from build123d import *

# Parameters (mm, degrees)
SKIZZE3_W                       = 11
SKIZZE3_H                       = 20
AUFSATZ_LINEAR_AUSTRAGEN1_DEPTH = 50
SKIZZE4_R                       = 2.375
SCHNITT_LINEAR_AUSTRAGEN1_DEPTH = 10
AUFSATZ_LINEAR_AUSTRAGEN2_DEPTH = 50
SKIZZE5_R                       = 2.3
SCHNITT_LINEAR_AUSTRAGEN2_DEPTH = 56.11862208
SKIZZE6_R                       = 3.75
SCHNITT_LINEAR_AUSTRAGEN3_DEPTH = 4.5
SKIZZE8_R                       = 4.25
SCHNITT_LINEAR_AUSTRAGEN4_DEPTH = 6.5
VERRUNDUNG1_R                   = 1
FASE1_SIZE                      = 0.75
VERRUNDUNG2_R                   = 2


with BuildPart() as part:
    # Skizze3 → Aufsatz-Linear austragen1 (new body)
    with BuildSketch(Plane.XY):
        with Locations((5.5, -10)):
            Rectangle(SKIZZE3_W, SKIZZE3_H)
    extrude(amount=-AUFSATZ_LINEAR_AUSTRAGEN1_DEPTH)

    # Skizze4 → Schnitt-Linear austragen1 (cut)
    with BuildSketch(Plane.ZY):
        with Locations(Location((-40, -7, 0), (0, 0, 270))):
            Circle(SKIZZE4_R)
        with Locations(Location((-10, -7, 0), (0, 0, 270))):
            Circle(SKIZZE4_R)
    extrude(amount=-SCHNITT_LINEAR_AUSTRAGEN1_DEPTH, mode=Mode.SUBTRACT)

    # Skizze7 → Aufsatz-Linear austragen2 (add)
    with BuildSketch(Plane.XY):
        Polygon((11, -13.5), (11, -6.5), (11.75, -7.25), (11.75, -12.75), align=None)
    extrude(amount=-AUFSATZ_LINEAR_AUSTRAGEN2_DEPTH)

    # Skizze5 → Schnitt-Linear austragen2 (cut, through all)
    with BuildSketch(Plane.ZY):
        with Locations(Location((-25, -10, 0), (0, 0, 270))):
            Circle(SKIZZE5_R)
    extrude(amount=-SCHNITT_LINEAR_AUSTRAGEN2_DEPTH, mode=Mode.SUBTRACT)

    # Skizze6 → Schnitt-Linear austragen3 (cut)
    with BuildSketch(Plane.ZY):
        with Locations(Location((-25, -10, 0), (0, 0, 270))):
            Circle(SKIZZE6_R)
    extrude(amount=-SCHNITT_LINEAR_AUSTRAGEN3_DEPTH, mode=Mode.SUBTRACT)

    # Skizze8 → Schnitt-Linear austragen4 (cut)
    with BuildSketch(Plane(origin=(11, 0, 0), x_dir=(0, 0, -1), z_dir=(1, 0, 0))):
        with Locations((25, -10)):
            Circle(SKIZZE8_R)
    extrude(amount=SCHNITT_LINEAR_AUSTRAGEN4_DEPTH, mode=Mode.SUBTRACT)

    # Verrundung1
    # the kernel refuses this fillet: 1 mm, written as the material it takes off along each edge
    with BuildSketch(Plane(origin=(11.75, -10, -25), x_dir=(0, 0.9561204309063354, -0.29297392649088017), z_dir=(0, 0.29297392649088017, 0.9561204309063354))) as verrundung1_piece_1:
        with BuildLine():
            CenterArc((5.218245837, 1), VERRUNDUNG1_R, 194.477512186, 75.522487814)
            Line((5.218245837, 0), (5.218245837, -0.02))
            Line((5.218245837, -0.02), (4.25, -0.02))
            Line((4.25, -0.02), (4.23, 0))
            ThreePointArc((4.23, 0), (4.23, 0.375), (4.230635083, 0.745))
            Line((4.230635083, 0.745), (4.25, 0.75))
        make_face()
    revolve(axis=Axis((11.75, -10, -25), (-1, 0, 0)), revolution_arc=145.927830349, mode=Mode.SUBTRACT)
    with BuildSketch(Plane(origin=(11.75, -10, -25), x_dir=(0, -0.9561204309062743, 0.292973926491079), z_dir=(0, -0.292973926491079, -0.9561204309062743))) as verrundung1_piece_2:
        with BuildLine():
            CenterArc((5.218245837, 1), VERRUNDUNG1_R, 194.477512186, 75.522487814)
            Line((5.218245837, 0), (5.218245837, -0.02))
            Line((5.218245837, -0.02), (4.25, -0.02))
            Line((4.25, -0.02), (4.23, 0))
            ThreePointArc((4.23, 0), (4.23, 0.375), (4.230635083, 0.745))
            Line((4.230635083, 0.745), (4.25, 0.75))
        make_face()
    revolve(axis=Axis((11.75, -10, -25), (-1, 0, 0)), revolution_arc=145.927830349, mode=Mode.SUBTRACT)

    # Fase1
    fase1_edges = [part.edges().sort_by_distance(p)[0] for p in [
        (5.5, -20, -50),
        (5.5, -20, 0),
        (5.5, 0, 0),
        (11, -20, -25),
        (0, -20, -25),
        (0, 0, -25),
        (11, 0, -25),
        (5.5, 0, -50),
    ]]
    chamfer(fase1_edges, length=FASE1_SIZE)

    # Verrundung2
    verrundung2_edges = [part.edges().sort_by_distance(p)[0] for p in [
        (11, -3.625, 0),
        (11, -3.625, -50),
        (11.375, -6.875, 0),
        (11.375, -13.125, 0),
        (11.75, -10, 0),
        (11.375, -6.875, -50),
        (11.75, -10, -50),
        (11.375, -13.125, -50),
        (0, -10, 0),
        (0, -10, -50),
        (11, -16.375, -50),
        (11, -16.375, 0),
    ]]
    fillet(verrundung2_edges, radius=VERRUNDUNG2_R)


solid = part.part
Input: part model. Units: mm. Frame: model coordinates. A direction names the side the tool comes from. Give positions to 0.01 mm unless a question says otherwise; leave off trailing zeros. Order: outer loops, then holes, each group sorted by start corner. A loop starts at its lowest first (then second) coordinate and runs counter-clockwise, first axis right, second up. Notation, with made-up numbers: (-13, 10.25) - (7, 10.25) arc R27 ccw to (7, 36.25) - close; hole circle Ø3 at (5.5, 20.25). An arc over 180 degrees is marked (long way). Answer as a JSON object with one key per item and string values. Group by question number.
Q1. Cut plane B-B, the plane x = 3.75. Output: boundary loops of the cut face in (y, z) (3 decimals), then the cut area to 3 significant figures.
Q2. First-contact query: pin 1 Ø1.5 at (y, z) = (-13, -27) entering from +X; pin 2 Ø1.4 at (y, z) = (-6.5, -10.5) entering from -X; pin 3 Ø6 at (y, z) = (-16, -17) entering from +X. Flat tips, straight axial feed; report the tip coordinate or a pass-through.
Q3. Mould query, pull axis Y, two halves, no side actions, for faces 1 (the face through (5, -20, -25)), 2 (the face through (10.815, -7.165, -49.43)), 3 (the face through (7.704, -8.175, -26.4)). Classes: pulls with the +Y half, pulls with the -Y half, needs draft (parallel to the pull), parting line crosses it, or undercut.
Q4. Cut plane D-D, the plane y = -10. Output: boundary loops of the cut face in (x, z).
Q5. Set-up query: faces 4 (the face through (4.93, -6.49, -42.32)), 5 (the face through (10.4, -16.2, -0.57)), 6 (the face through (10.4, -3.7, -0.57)). Return all of +Z, -Z, +X, -X, +Y, -Y with unobstructed straight access to the full face (end or side cutting, diameter ignored); none if empty.
Q6. Line query: probe 1 along X at (y, z) = (-17.5, -43.5); probe 2 along Z at (x, y) = (1.45, -10); probe 3 along Z at (x, y) = (10.5, -9.5) (3 decimals). Output: solid intervals per line, ascending.
Q7. Cut plane A-A, the plane z = -25. Output: boundary loops of the cut face in (x, y), then the cut area to 3 significant figures.
Q8. Cut plane C-C, the plane y = -2. Output: boundary loops of the cut face in (x, z), then the cut area to 3 significant figures.
Results:
{
 "1": {"outline": "(-20, -49.25) - (-19.25, -50) - (-0.75, -50) - (0, -49.25) - (0, -0.75) - (-0.75, 0) - (-19.25, 0) - (-20, -0.75) - close; hole circle Ø7.5 at (-10, -25); hole circle Ø4.75 at (-7, -40); hole circle Ø4.75 at (-7, -10)", "area": "919 mm^2"},
 "2": {"pin 1": "x = 11.12", "pin 2": "x = 10", "pin 3": "x = 11.5"},
 "3": {"face 1": "pulls with the -Y half", "face 2": "pulls with the +Y half", "face 3": "undercut"},
 "4": {"outline": "(0, -48) arc R2 ccw to (2, -50) - (9.75, -50) arc R2 ccw to (11.75, -48) - (11.75, -30.22) arc R1 ccw to (11, -29.25) - (11, -27.3) - (4.5, -27.3) - (4.5, -28.75) - (0, -28.75) - close; (0, -21.25) - (4.5, -21.25) - (4.5, -22.7) - (11, -22.7) - (11, -20.75) arc R1 ccw to (11.75, -19.78) - (11.75, -2) arc R2 ccw to (9.75, 0) - (2, 0) arc R2 ccw to (0, -2) - close"},
 "5": {"face 4": "-X", "face 5": "+Z, +X, -Y", "face 6": "+Z, +X, +Y"},
 "6": {"probe 1": "0 to 11", "probe 2": "-49.92 to -28.75, -21.25 to -0.08", "probe 3": "-49.854 to -27.245, -22.755 to -0.146"},
 "7": {"outline": "(0, -19.25) - (0.75, -20) - (10.25, -20) - (11, -19.25) - (11, -12.3) - (4.5, -12.3) - (4.5, -13.75) - (0, -13.75) - close; (0, -6.25) - (4.5, -6.25) - (4.5, -7.7) - (11, -7.7) - (11, -0.75) - (10.25, 0) - (0.75, 0) - (0, -0.75) - close", "area": "155 mm^2"},
 "8": {"outline": "(0, -48) arc R2 ccw to (2, -50) - (9, -50) arc R2 ccw to (11, -48) - (11, -2) arc R2 ccw to (9, 0) - (2, 0) arc R2 ccw to (0, -2) - close", "area": "547 mm^2"}
}
